The figure shows three views and two pictorial views of one solid part (mm, origin at its lowest corner). Answer the questions. Coordinates: 2 decimals unless noted, no trailing zeros. Answer in a Markdown table with one row per item.
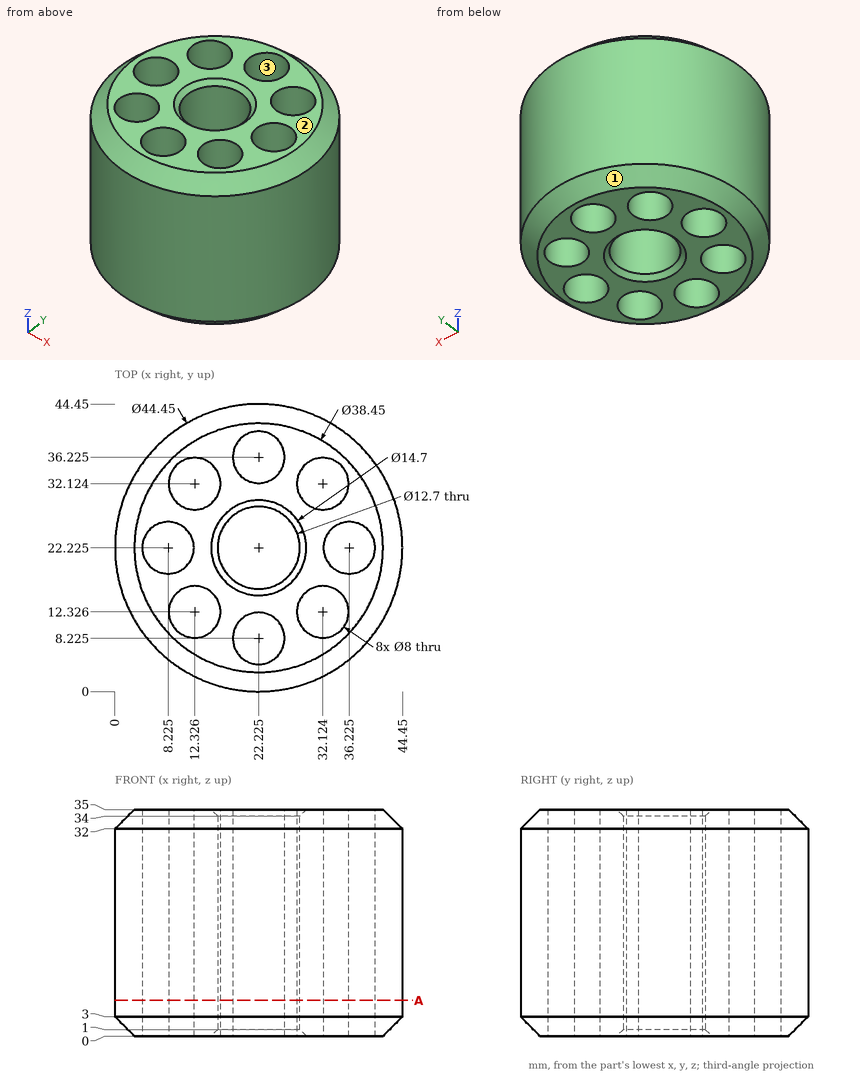
Item 1: Determine the mould class of the marked faces 1, 2 and 3 for opening direction X: +X half, -X half, draft (parallel to the pull), parting line (faces both ways), or undercut.
Findings below:
| item | result |
|---|---|
| face 1 | parting line |
| face 2 | draft |
| face 3 | undercut |
Item 2: Find the intervals of material crossed by probe 1 along Y at (x, z) = (32, 4) (1 decimal); probe 2 along X at (y, z) = (30.5, 15); probe 3 along Y at (x, z) = (21.5, 18), in increasing order.
Findings below:
| item | result |
|---|---|
| probe 1 | y = 2.3 to 8.3, 16.3 to 28.1, 36.1 to 42.2 |
| probe 2 | x = 1.6 to 8.67, 15.98 to 28.47, 35.78 to 42.85 |
| probe 3 | y = 0.01 to 4.29, 12.16 to 15.92, 28.53 to 32.29, 40.16 to 44.44 |
Item 3: A cutting plane is placed at A-A, the plane z = 5.5. Count the separate pieces of the cut face and the enclosed holes in it, plus the area to 3 significant figures.
Findings below:
| item | result |
|---|---|
| separate pieces | 1 |
| enclosed holes | 9 |
| area | 1,020 mm2 |
Item 4: Flat-ended cylindrical pins translate along their axes: pin 1 Ø2 at (y, z) = (5, 19.5) entering from -X (1 decimal); pin 2 Ø7 at (x, y) = (12.33, 12.33) entering from -Z; pin 3 Ø1.5 at (y, z) = (34, 12) entering from -X; pin 4 Ø12 at (y, z) = (9, 27) entering from +X. Find the tip coordinate at first contact, or state that the pin passes through.
Findings below:
| item | result |
|---|---|
| pin 1 | stops at x = 7 |
| pin 2 | passes through |
| pin 3 | stops at x = 2.93 |
| pin 4 | stops at x = 43.24 |
